Check sheet for the modelled part. Datum: model origin and axes. Units: mm. A direction names the side the tool comes from. Round coordinates to 2 decimals unless told otherwise and drop trailing zeros. Order: outer loops, then holes, each group sorted by start corner. A loop starts at its lowest first (then second) coordinate and runs counter-clockwise, first axis right, second up.
(1) Thickness scan on probe 1 along Y at (x, z) = (-7, 28.5); probe 2 along X at (y, z) = (-33.5, 23.5); probe 3 along X at (y, z) = (-8, 12.5). Record the ranges inside material, lowest first.
(2) Mould release check, pull along Y, two halves, no side actions. Record for faces 1 (the flat face through (4, -2.54, 26)), 2 (the flat face through (4, -149.86, 25)), 3 (the flat face through (15.3, -73.9, 18.2)), 4 (the flat face through (4, 0, 25)): released by +Y, released by -Y, zero draft, split by the parting line, or undercut.
(3) Sectioned sample at D-D, the plane y = -59.5. Enter the section's corners in (x, z).
(4) Sectioned sample at B-B, the plane x = -2.5. Enter the section's corners in (y, z).
(5) Tool access check on faces 5 (the flat face through (-12.934, -73.881, 20.306)), 6 (the flat face through (16.707, -96.28, 17.812)), 7 (the flat face through (-16.516, -96.28, 28.325)), 8 (the flat face through (-11, -74, 22)). Record the directions out of +Z, -Z, +X, -X, +Y, -Y that give a thin tool (end or side, any length) a straight path to the whole face; none if there is none.
(6) Depth check by flat-ended pin: pin 1 (2 mm diameter, centred on x = -19.5, y = -60, fed in from -Z); pin 2 (1 mm diameter, centred on x = -19.5, y = -47.5, fed in from +Z); pin 3 (12 mm diameter, centred on x = 9, z = 19.5, fed in from +Y); pin 4 (1.5 mm diameter, centred on y = -112, z = 28.5, fed in from +X). Enter the tip coordinate at first touch or a pass-through.
(7) Sectioned sample at C-C, the plane z = 10. Enter the section's corners in (x, y).
(8) Sectioned sample at A-A, the plane y = -90.5. Enter the section's corners in (x, z).
```python
from build123d import *

# Parameters (mm, degrees)
F1_DEPTH = 149.86
F3_T     = -2.54
F2_W     = 34.298644
F2_H     = 15.946299
F4_DEPTH = 94.234


with BuildPart() as f1:
    # F0 (on Front) → F1 (new body)
    with BuildSketch(Plane.XZ):
        Polygon((-25.51176, 40.050719), (0, 0), (33.741359, 32.369759), align=None)
    extrude(amount=F1_DEPTH)

    # F3
    f3_openings = [f1.faces().sort_by_distance(p)[0] for p in [
        (4.114799, -74.93, 36.210239),
    ]]
    offset(amount=F3_T, openings=f3_openings)

    # F2 (on face) → F4 (cut)
    with BuildSketch(Plane(origin=(4.684349, 0, 36.136408), x_dir=(0.991703, 0, -0.128554), z_dir=(0.128554, 0, 0.991703))):
        with Locations((-2.870781, -96.167914)):
            Rectangle(F2_W, F2_H)
    extrude(amount=-F4_DEPTH, mode=Mode.SUBTRACT)


solid = f1.part
```
Derived:
1. probe 1: y = -149.86 to -147.32, -2.54 to 0
1. probe 2: x = -14.97 to -11.96, 20.83 to 24.5
1. probe 3: x = -7.96 to -4.95, 9.36 to 13.03
2. face 1: undercut
2. face 2: released by -Y
2. face 3: undercut
2. face 4: released by +Y
3. outline: (-25.51, 40.05) - (0, 0) - (33.74, 32.37) - (30.51, 32.79) - (0.48, 3.98) - (-22.23, 39.63) - close
4. outline: (-149.86, 3.92) - (-104.14, 3.92) - (-104.14, 8.65) - (-147.32, 8.65) - (-147.32, 37.07) - (-149.86, 37.07) - close; (-88.19, 3.92) - (0, 3.92) - (0, 37.07) - (-2.54, 37.07) - (-2.54, 8.65) - (-88.19, 8.65) - close
5. face 5: -Z, -X, +Y, -Y
5. face 6: +Z, -X
5. face 7: -Z
5. face 8: +Z
6. pin 1: stops at z = 29.04
6. pin 2: stops at z = 36.13
6. pin 3: stops at y = 0
6. pin 4: stops at x = 30.49
7. outline: (-6.37, -149.86) - (10.42, -149.86) - (10.42, -104.14) - (6.75, -104.14) - (6.75, -147.32) - (-3.36, -147.32) - (-3.36, -104.14) - (-6.37, -104.14) - close; (-6.37, -88.19) - (-3.36, -88.19) - (-3.36, -2.54) - (6.75, -2.54) - (6.75, -88.19) - (10.42, -88.19) - (10.42, 0) - (-6.37, 0) - close
8. outline: (-25.51, 40.05) - (-16.77, 26.33) - (-16.26, 30.26) - (-22.23, 39.63) - close; (16.44, 15.77) - (33.74, 32.37) - (30.51, 32.79) - (16.96, 19.79) - close
